Part model, mm, in its own coordinate system. A direction names the side the tool comes from. Give positions to 0.01 mm unless a question says otherwise; leave off trailing zeros. Write each loop counter-clockwise with the first axis right and the second up, starting at its lowest first coordinate (ties: lowest second). Pieces come first, ordered by that corner, then holes. Notation, with made-up numbers: M 66,-28 L 123,-28 A20 cw 123,-13 Z; hole C -24,5 d7. An arc over 180 degrees is marked long. Answer as CSV lines item,"result". Start each with the question number.
Item 1: Band-saw the part on B-B, the plane x = 21.9. List the corners of the cut face in (y, z).
Item 2: Band-saw the part on C-C, the plane y = 9.5. List the corners of the cut face in (x, z) (3 decimals).
Item 3: Pin check, flat tips, straight feed: pin 1 (0.5 mm diameter, centred on y = 2, z = 3, fed in from +X); pin 2 (3 mm diameter, centred on y = 4, z = -5.5, fed in from -X); pin 3 (1.5 mm diameter, centred on x = 3, y = 7.5, fed in from -Z); pin 4 (1.4 mm diameter, centred on x = -10.62, z = -23.5, fed in from -Y). Stop position of each tip, or through.
Item 4: Wall check: L1, parallel to Z at x = 25, y = 7.75; L2, parallel to X at y = 7.25, z = -13.25; L3, parallel to Z at x = 18, y = 7. Give the ranges that are in metal, low to high. Write a range as from..to.
Item 5: 3-axis set-ups, long thin cutter, end or side, ignore diameter. For faces 1 (the flat face through (31, 5, -10.174)), 2 (the flat face through (-9.117, 5, -22)), 3 (the flat face through (1.3, 7.4, -20.5)), 4 (the flat face through (1.3, 5, -3)): which of +Z, -Z, +X, -X, +Y, -Y reach the whole face in a straight line?
Item 6: Band-saw the part on A-A, the plane z = -16.75. List the corners of the cut face in (x, y).
Item 7: Band-saw the part on D-D, the plane x = 34. Count the separate pieces of the cut face and the enclosed holes in it, then the cut area to 3 significant figures.
from build123d import *

# Parameters (mm, degrees)
CROQUIS1_R              = 1.55
SALIENTE_EXTRUIR1_DEPTH = 10.5
CROQUIS2_R              = 1.2
SALIENTE_EXTRUIR2_DEPTH = 4.3
SALIENTE_EXTRUIR6_DEPTH = 4.3
SALIENTE_EXTRUIR7_DEPTH = 7.5
CROQUIS5_R              = 1.8
CORTAR_EXTRUIR1_DEPTH   = 1.5
CROQUIS6_W              = 9.1
CROQUIS6_H              = 0.8
SALIENTE_EXTRUIR8_DEPTH = 6.2
CORTAR_EXTRUIR2_DEPTH   = 7.2


with BuildPart() as part:
    # Croquis1 → Saliente-Extruir1 (new body)
    with BuildSketch(Plane(origin=(0, 0, 0), x_dir=(1, 0, 0), z_dir=(0, 1, 0))):
        with BuildLine():
            Line((3, 0), (25, 0))
            ThreePointArc((25, 0), (27.121320344, 0.878679656), (28, 3))
            Line((28, 3), (28, 13))
            ThreePointArc((28, 13), (27.121320344, 15.121320344), (25, 16))
            Line((25, 16), (3, 16))
            ThreePointArc((3, 16), (0.878679656, 15.121320344), (0, 13))
            Line((0, 13), (0, 3))
            ThreePointArc((0, 3), (0.878679656, 0.878679656), (3, 0))
        make_face()
        with Locations((25, 13.25)):
            Circle(CROQUIS1_R, mode=Mode.SUBTRACT)
        Polygon((1.3, 3.525), (2.075, 4.3), (3.925, 4.3), (4.7, 3.525), (4.7, 1.975), (3.925, 1.2), (2.075, 1.2), (1.3, 1.975), (1.3, 2.75), align=None, mode=Mode.SUBTRACT)
    extrude(amount=SALIENTE_EXTRUIR1_DEPTH)

    # Croquis2 → Saliente-Extruir2 (add)
    with BuildSketch(Plane(origin=(0, 3.1, 0), x_dir=(1, 0, 0), z_dir=(0, 1, 0))):
        with BuildLine():
            Line((-12.117246013, 20), (15.502753987, 20))
            ThreePointArc((15.502753987, 20), (15.795636527, 19.916267232), (16, 19.69037582))
            Line((16, 19.69037582), (16, 16))
            Line((16, 16), (17, 16))
            Line((17, 16), (17, 20))
            ThreePointArc((17, 20), (16.707106781, 20.707106781), (16, 21))
            Line((16, 21), (-9.117246013, 21))
            Line((-9.117246013, 21), (-9.117246013, 23.5))
            ThreePointArc((-9.117246013, 23.5), (-10.617246013, 25), (-12.117246013, 23.5))
            Line((-12.117246013, 23.5), (-12.117246013, 21))
            Line((-12.117246013, 21), (-12.117246013, 20))
        make_face()
        with Locations((-10.617246013, 23.5)):
            Circle(CROQUIS2_R, mode=Mode.SUBTRACT)
    extrude(amount=SALIENTE_EXTRUIR2_DEPTH)

    # Croquis3 → Saliente-Extruir6 (add)
    with BuildSketch(Plane(origin=(0, 3.1, 0), x_dir=(1, 0, 0), z_dir=(0, 1, 0))):
        with BuildLine():
            Line((4.579945188, 19.96820969), (5.178103837, 19.958862719))
            ThreePointArc((5.178103837, 19.958862719), (5.85002436, 19.513199542), (6.110061503, 18.75))
            Line((6.110061503, 18.75), (6.110061503, 16))
            Line((6.110061503, 16), (3.610061503, 16))
            Line((3.610061503, 16), (3.610061503, 18.75))
            ThreePointArc((3.610061503, 18.75), (3.882143972, 19.52857389), (4.579945188, 19.96820969))
        make_face()
    extrude(amount=SALIENTE_EXTRUIR6_DEPTH)

    # Croquis4 → Saliente-Extruir7 (add)
    with BuildSketch(Plane(origin=(0, 1.5, 0), x_dir=(1, 0, 0), z_dir=(0, 1, 0))):
        Polygon((15, 0), (15, -2.7), (26, -2.7), (26, -3.5), (15, -3.5), (14.2, -3.5), (14.2, 0), align=None)
    extrude(amount=SALIENTE_EXTRUIR7_DEPTH)

    # Croquis5 → Cortar-Extruir1 (cut)
    with BuildSketch(Plane.XY.offset(3.5)):
        with Locations((21.9, 5.25)):
            Circle(CROQUIS5_R)
        with BuildLine():
            Line((26, 1.5), (18.3, 1.5))
            Line((18.3, 1.5), (18.3, 2.1))
            Line((18.3, 2.1), (25.646446609, 2.1))
            ThreePointArc((25.646446609, 2.1), (25.896446609, 2.203553391), (26, 2.453553391))
            Line((26, 2.453553391), (26, 8.046446609))
            ThreePointArc((26, 8.046446609), (25.896446609, 8.296446609), (25.646446609, 8.4))
            Line((25.646446609, 8.4), (18.3, 8.4))
            Line((18.3, 8.4), (18.3, 9))
            Line((18.3, 9), (27.293222539, 9))
            Line((27.293222539, 9), (27.293222539, 1.5))
            Line((27.293222539, 1.5), (26, 1.5))
        make_face()
    extrude(amount=-CORTAR_EXTRUIR1_DEPTH, mode=Mode.SUBTRACT)

    # Croquis6 → Saliente-Extruir8 (add)
    with BuildSketch(Plane(origin=(0, 2.15, 0), x_dir=(1, 0, 0), z_dir=(0, 1, 0))):
        with Locations((32.55, 10.574019752)):
            Rectangle(CROQUIS6_W, CROQUIS6_H)
        with Locations((32.55, 5.301623485)):
            Rectangle(CROQUIS6_W, CROQUIS6_H)
    extrude(amount=SALIENTE_EXTRUIR8_DEPTH)

    # Croquis7 → Cortar-Extruir2 (cut)
    with BuildSketch(Plane(origin=(0, 0, -10.974019752), x_dir=(-1, 0, 0), z_dir=(0, 0, -1))):
        with BuildLine():
            Line((-37.1, 2.15), (-30.7, 2.15))
            Line((-30.7, 2.15), (-30.7, 2.85))
            Line((-30.7, 2.85), (-36.746446609, 2.85))
            ThreePointArc((-36.746446609, 2.85), (-36.996446609, 2.953553391), (-37.1, 3.203553391))
            Line((-37.1, 3.203553391), (-37.1, 7.296446609))
            ThreePointArc((-37.1, 7.296446609), (-36.996446609, 7.546446609), (-36.746446609, 7.65))
            Line((-36.746446609, 7.65), (-30.7, 7.65))
            Line((-30.7, 7.65), (-30.7, 8.35))
            Line((-30.7, 8.35), (-37.1, 8.35))
            Line((-37.1, 8.35), (-38.596530357, 8.35))
            Line((-38.596530357, 8.35), (-38.596530357, 2.85))
            Line((-38.596530357, 2.85), (-38.596530357, 2.15))
            Line((-38.596530357, 2.15), (-37.1, 2.15))
        make_face()
        with BuildLine():
            add(Edge.make_bspline(
                [(-32.392984362, 5.25), (-32.743324346, 3.873805387), (-34.382207103, 4.479328863), (-34.892984362, 5.25)],
                knots=[0, 0, 0, 0, 1, 1, 1, 1], degree=3))
            add(Edge.make_bspline(
                [(-32.392984362, 5.25), (-32.743324346, 6.626194613), (-34.382207103, 6.020671137), (-34.892984362, 5.25)],
                knots=[0, 0, 0, 0, 1, 1, 1, 1], degree=3))
        make_face()
    extrude(amount=-CORTAR_EXTRUIR2_DEPTH, mode=Mode.SUBTRACT)


solid = part.part
Output:
1,outline,"M 0,-16 L 10.5,-16 L 10.5,0 L 0,0 Z; M 2.1,2.7 L 3.45,2.7 L 3.45,3.5 L 2.1,3.5 Z; M 7.05,2.7 L 8.4,2.7 L 8.4,3.5 L 7.05,3.5 Z"
2,outline,"M 0,-13 A3 ccw 3,-16 L 25,-16 A3 ccw 28,-13 L 28,-3 A3 ccw 25,0 L 3,0 A3 ccw 0,-3 Z; hole M 1.3,-3.525 L 2.075,-4.3 L 3.925,-4.3 L 4.7,-3.525 L 4.7,-1.975 L 3.925,-1.2 L 2.075,-1.2 L 1.3,-1.975 Z; hole C 25,-13.25 d3.1"
3,pin 1,"x = 25.94"
3,pin 2,"x = 0"
3,pin 3,"z = -21"
3,pin 4,"through"
4,L1,"-16..-14.8, -11.7..0, 2.7..3.5"
4,L2,"0.01..23.45, 26.55..27.99"
4,L3,"-16..0, 2.7..3.5"
5,face 1,"+X, +Y, -Y"
5,face 2,"-Z, +X, +Y, -Y"
5,face 3,"-Z, +X, -X, +Y"
5,face 4,"+Y, -Y"
6,outline,"M 3.61,3.1 L 6.11,3.1 L 6.11,7.4 L 3.61,7.4 Z; M 16,3.1 L 17,3.1 L 17,7.4 L 16,7.4 Z"
7,separate pieces,"4"
7,enclosed holes,"0"
7,area,"5.47 mm²"
